Build history of the part. All positions in model axes, mm. Round coordinates to 2 decimals unless told otherwise and drop trailing zeros. Write each loop counter-clockwise with the first axis right and the second up, starting at its lowest first coordinate (ties: lowest second). Pieces come first, ordered by that corner, then holes. Notation, with made-up numbers: (1.25, 13) -> (47.25, 13) arc R4 ccw to (47.25, 17) -> close; hole circle Ø11 at (25, 82.25). An arc over 180 degrees is marked (long way). Answer in a Markdown table with one row per item.
```python
from build123d import *

# Parameters (mm, degrees)
SKETCH_2_W          = 250
SKETCH_2_H          = 150
EXTRUDE_1_DEPTH     = 80.07
SKETCH_6_R          = 7.5
CUT_EXTRUDE_1_DEPTH = 20
SKETCH_7_W          = 250
SKETCH_7_H          = 150
EXTRUDE_2_DEPTH     = 21.15
SKETCH_13_R         = 2.5
EXTRUDE_4_DEPTH     = 20
SKETCH_15_R         = 2.5
EXTRUDE_5_DEPTH     = 20


with BuildPart() as part:
    # 草图2 → 凸台-拉伸1 (new body)
    with BuildSketch(Plane(origin=(0, 0, 0), x_dir=(1, 0, 0), z_dir=(0, 1, 0))):
        Rectangle(SKETCH_2_W, SKETCH_2_H)
    extrude(amount=EXTRUDE_1_DEPTH)

    # 草图6 → 切除-拉伸1 (cut)
    with BuildSketch(Plane(origin=(0, 0, -75), x_dir=(-1, 0, 0), z_dir=(0, 0, -1))):
        with Locations((-22.5, 40.035)):
            Circle(SKETCH_6_R)
        with Locations((22.5, 40.035)):
            Circle(SKETCH_6_R)
    extrude(amount=-CUT_EXTRUDE_1_DEPTH, mode=Mode.SUBTRACT)

    # 草图7 → 凸台-拉伸2 (add)
    with BuildSketch(Plane(origin=(0, 80.07, 0), x_dir=(1, 0, 0), z_dir=(0, 1, 0))):
        Rectangle(SKETCH_7_W, SKETCH_7_H)
    extrude(amount=EXTRUDE_2_DEPTH)

    # 草图13 → 凸台-拉伸4 (add)
    with BuildSketch(Plane(origin=(0, 101.22, 0), x_dir=(1, 0, 0), z_dir=(0, 1, 0))):
        with Locations(Location((11, 58, 0), (0, 0, 270))):
            Circle(SKETCH_13_R)
    extrude(amount=EXTRUDE_4_DEPTH)

    # 草图15 → 凸台-拉伸5 (add)
    with BuildSketch(Plane(origin=(0, 101.22, 0), x_dir=(1, 0, 0), z_dir=(0, 1, 0))):
        with Locations(Location((50, -4, 0), (0, 0, 270))):
            Circle(SKETCH_15_R)
        with Locations(Location((-50, -4, 0), (0, 0, 90))):
            Circle(SKETCH_15_R)
    extrude(amount=EXTRUDE_5_DEPTH)


solid = part.part
```
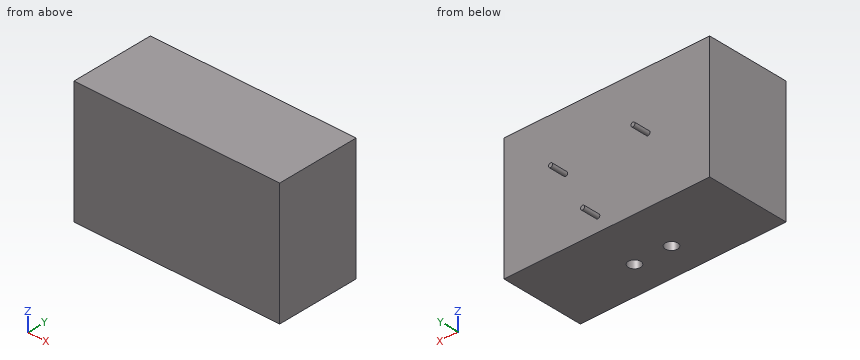
Q1. Saw through at B-B on z = -15.5. Write the cut outline in (x, y).
A:
| item | result |
|---|---|
| outline | (-125, 0) -> (125, 0) -> (125, 101.22) -> (-125, 101.22) -> close |
Q2. Saw through at A-A on x = -22.5. Write the cut outline in (y, z) (3 decimals).
A:
| item | result |
|---|---|
| outline | (0, -75) -> (32.535, -75) -> (32.535, -55) -> (47.535, -55) -> (47.535, -75) -> (101.22, -75) -> (101.22, 75) -> (0, 75) -> close |
Q3. Saw through at C-C on y = 105. Write the cut outline in (x, z).
A:
| item | result |
|---|---|
| outline | circle Ø5 at (-50, 4); circle Ø5 at (11, -58); circle Ø5 at (50, 4) |
Q4. Wall check: line 1 (Y direction, x = -22.5, z = -69.75) (3 decimals); line 2 (Y direction, x = -74, z = -32). Give the ranges that are in metal, low to high. Write a range as [from, to].
A:
| item | result |
|---|---|
| line 1 | [0, 32.535], [47.535, 101.22] |
| line 2 | [0, 101.22] |
Q5. Saw through at D-D on x = 27. Write the cut outline in (y, z) (3 decimals).
A:
| item | result |
|---|---|
| outline | (0, -75) -> (34.035, -75) -> (34.035, -55) -> (46.035, -55) -> (46.035, -75) -> (101.22, -75) -> (101.22, 75) -> (0, 75) -> close |
Q6. Drop flat-ended pins along their axis: P1, Ø8, axis at x = -97, z = -1, coming from the +Y side; P2, Ø12, axis at x = 22.5, y = 40.035, coming from the -Z side; P3, Ø10, axis at x = 3, z = -56.5, coming from the -Y side. Give the stop position or say it passes through.
A:
| item | result |
|---|---|
| P1 | y = 101.22 |
| P2 | z = -55 |
| P3 | y = 0 |
